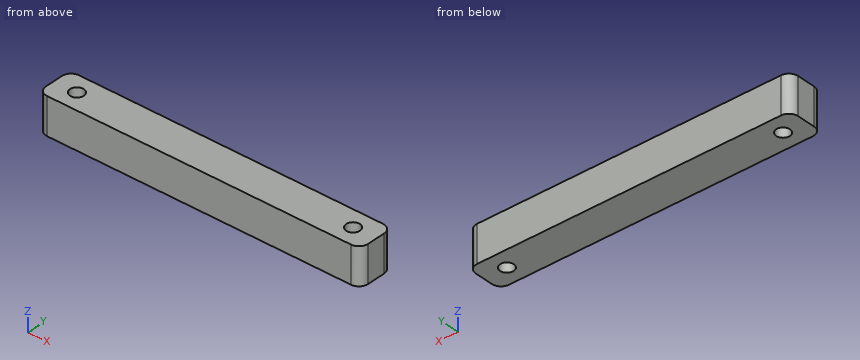
from build123d import *

# Parameters (mm, degrees)
SKETCH_1_W      = 70
SKETCH_1_H      = 8
SKETCH_1_R      = 1.5
EXTRUDE_1_DEPTH = 8
FILLET_1_R      = 2


with BuildPart() as part:
    # 草图1 → 凸台-拉伸1 (new body)
    with BuildSketch(Plane.XY):
        with Locations((35, -4)):
            Rectangle(SKETCH_1_W, SKETCH_1_H)
        with Locations((5, -4)):
            Circle(SKETCH_1_R, mode=Mode.SUBTRACT)
        with Locations(Location((65, -4, 0), (0, 0, 180))):
            Circle(SKETCH_1_R, mode=Mode.SUBTRACT)
    extrude(amount=EXTRUDE_1_DEPTH)

    # 圆角1
    fillet_1_edges = [part.edges().sort_by_distance(p)[0] for p in [
        (0, 0, 4),
        (70, 0, 4),
        (70, -8, 4),
        (0, -8, 4),
    ]]
    fillet(fillet_1_edges, radius=FILLET_1_R)


solid = part.part
Geometry check sheet. Reference: the model listing, model coordinates, mm. Give positions to 0.01 mm unless a question says otherwise; leave off trailing zeros. Order: outer loops, then holes, each group sorted by start corner. A loop starts at its lowest first (then second) coordinate and runs counter-clockwise, first axis right, second up. Notation, with made-up numbers: (41.25, 86.5) - (90.25, 86.5) arc R18 cw to (90.25, 96.5) - close; hole circle Ø9 at (7.5, 22.5). An arc over 180 degrees is marked (long way). Answer as a JSON object with one key per item and string values.
(1) Cross-section at B-B (y = -4). Record the cut outline in (x, z).
Report:
{"outline": "(0, 0) - (3.5, 0) - (3.5, 8) - (0, 8) - close; (6.5, 0) - (63.5, 0) - (63.5, 8) - (6.5, 8) - close; (66.5, 0) - (70, 0) - (70, 8) - (66.5, 8) - close"}
(2) Material ranges on line 1 (Y direction, x = 5, z = 4); line 2 (X direction, y = -2.75, z = 7.5); line 3 (X direction, y = -4.5, z = 7.5), recorded low to high.
Report:
{"line 1": "-8 to -5.5, -2.5 to 0", "line 2": "0 to 4.17, 5.83 to 64.17, 65.83 to 70", "line 3": "0 to 3.59, 6.41 to 63.59, 66.41 to 70"}
(3) Cross-section at A-A (x = 5). Record the cut outline in (y, z), then the cut area to 3 significant figures.
Report:
{"outline": "(-8, 0) - (-5.5, 0) - (-5.5, 8) - (-8, 8) - close; (-2.5, 0) - (0, 0) - (0, 8) - (-2.5, 8) - close", "area": "40.0 mm^2"}
(4) Depth check by flat-ended pin: pin 1 Ø1 at (y, z) = (-1, 7) entering from -X; pin 2 Ø4 at (x, y) = (65, -4) entering from -Z. Enter the tip coordinate at first touch or a pass-through.
Report:
{"pin 1": "x = 0.06", "pin 2": "z = 0"}
(5) Cross-section at C-C (z = 4). Record the cut outline in (x, y), then the cut area to 3 significant figures.
Report:
{"outline": "(0, -6) arc R2 ccw to (2, -8) - (68, -8) arc R2 ccw to (70, -6) - (70, -2) arc R2 ccw to (68, 0) - (2, 0) arc R2 ccw to (0, -2) - close; hole circle Ø3 at (5, -4); hole circle Ø3 at (65, -4)", "area": "542 mm^2"}
